Study the drawing (mm; zero at the part's minimum x, y, z) and answer. A direction names the side the tool comes from. Round coordinates to 2 decimals unless told otherwise and drop trailing zeros. Write each loop counter-clockwise with the first axis right and the second up, starting at its lowest first coordinate (ties: lowest second). Pieces come first, ordered by that corner, then holes. Notation, with made-up numbers: (-7.75, 24.25) -> (39.25, 24.25) arc R26 ccw to (39.25, 47.25) -> close; hole circle Ø3 at (-20.5, -16.75). An arc over 180 degrees is marked (long way). Return JSON: item names as keys, results as strings.
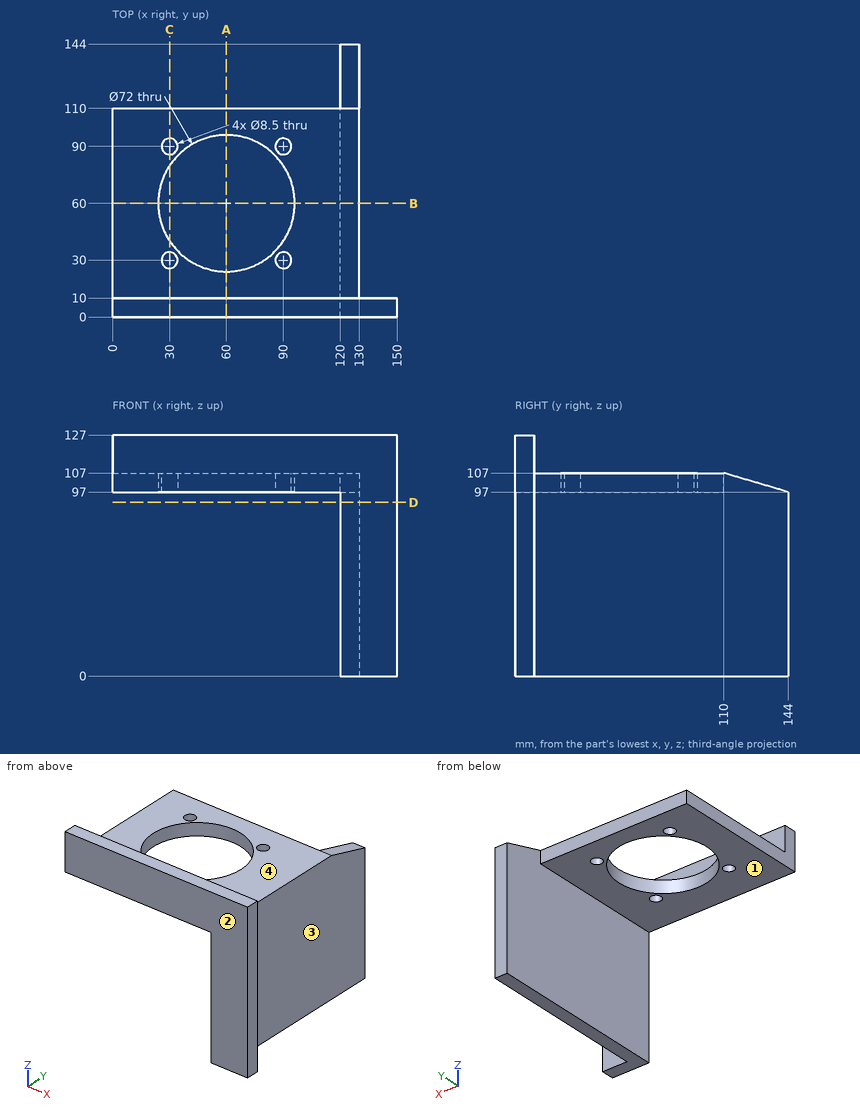
Item 1: Straight lines are drawn through the part: L1, parallel to Y at x = 60, z = 100.75; L2, parallel to Y at x = 30, z = 102.5; L3, parallel to Z at x = 124.5, y = 24. For each, find the intervals that lie inside material, in ascending order. Write a range as [from, to].
Worked answers:
{"L1": "y = [0, 24], [96, 110]", "L2": "y = [0, 25.75], [34.25, 40.1], [79.9, 85.75], [94.25, 110]", "L3": "z = [0, 107]"}
Item 2: Flat-ended cylindrical pins translate along their axes: pin 1 (3 mm diameter, centred on x = 110.5, y = 78, fed in from -Z); pin 2 (11 mm diameter, centred on x = 78, z = 102.5, fed in from +Y); pin 3 (3 mm diameter, centred on y = 92, z = 71.5, fed in from -X). Find the tip coordinate at first contact, or state that the pin passes through.
Worked answers:
{"pin 1": "stops at z = 97", "pin 2": "stops at y = 110", "pin 3": "stops at x = 120"}
Item 3: Section C-C (x = 30) is taken. Give the vertices of the cut face in (y, z), then the cut area to 3 significant figures.
Worked answers:
{"outline": "(0, 97) -> (25.75, 97) -> (25.75, 107) -> (10, 107) -> (10, 127) -> (0, 127) -> close; (34.25, 97) -> (40.1, 97) -> (40.1, 107) -> (34.25, 107) -> close; (79.9, 97) -> (85.75, 97) -> (85.75, 107) -> (79.9, 107) -> close; (94.25, 97) -> (110, 97) -> (110, 107) -> (94.25, 107) -> close", "area": "732 mm2"}
Item 4: Section A-A (x = 60) is taken. Give the vertices of the cut face in (y, z).
Worked answers:
{"outline": "(0, 97) -> (24, 97) -> (24, 107) -> (10, 107) -> (10, 127) -> (0, 127) -> close; (96, 97) -> (110, 97) -> (110, 107) -> (96, 107) -> close"}
Item 5: Section B-B (y = 60) is taken. Give the vertices of the cut face in (x, z).
Worked answers:
{"outline": "(0, 97) -> (24, 97) -> (24, 107) -> (0, 107) -> close; (96, 97) -> (120, 97) -> (120, 0) -> (130, 0) -> (130, 107) -> (96, 107) -> close"}
Item 6: Section D-D (z = 91.5) is taken. Give the vertices of the cut face in (x, y).
Worked answers:
{"outline": "(120, 0) -> (150, 0) -> (150, 10) -> (130, 10) -> (130, 144) -> (120, 144) -> close"}
Item 7: A tool of negligible diameter and unlimited length cuts with its end or side. For the marked faces 3 and 4, from which of +Z, -Z, +X, -X, +Y, -Y can it reach the whole face along a straight path? Write none if from no direction.
Worked answers:
{"face 3": "+Z, -Z, +X, +Y", "face 4": "+Z, +X, -X, +Y"}
Item 8: For a pull along Y with two mould halves and no side action, classify the marked faces 1 and 2 as released by +Y, released by -Y, zero draft, split by the parting line, or undercut.
Worked answers:
{"face 1": "zero draft", "face 2": "released by -Y"}
